Geometry check sheet. Reference: the model listing, model coordinates, mm. A direction names the side the tool comes from. Give positions to 0.01 mm unless a question says otherwise; leave off trailing zeros. Order: outer loops, then holes, each group sorted by start corner. A loop starts at its lowest first (then second) coordinate and runs counter-clockwise, first axis right, second up. Notation, with made-up numbers: M 73,5.5 L 93,5.5 A23 cw 93,43.5 Z; hole C 63.5,-26.5 d7. An arc over 180 degrees is marked long. Put each result on its own line as item: value. Start each with the question number.
Q1. Material ranges on L1, parallel to X at y = 17.75, z = 20; L2, parallel to Y at x = 45, z = 7; L3, parallel to Z at x = 37.5, y = 19, recorded low to high.
Q2. Section check A-A on y = 18. Record the cut outline in (x, z).
Q3. Section check C-C on z = -14.5. Record the cut outline in (x, y).
Q4. Mould release check, pull along Y, two halves, no side actions. Record for faces 4 (the cylindrical face through (8.628, 14.435, -21.014)), 5 (the flat face through (26, 24.7, -11)), 6 (the flat face through (24, 3, 32)): +Y half, -Y half, draft (parallel to the pull), parting line (faces both ways), or undercut.
Q5. Section check B-B on x = 22.5. Record the cut outline in (y, z).
Q6. Access from +Z, -Z, +X, -X, +Y, -Y to the whole of each face (thin tool, end or side, straight path). Record for faces 1 (the flat face through (3.4, 13, 17)), 2 (the flat face through (25, 1.4, 17)), 3 (the flat face through (49.4, 13, 17)).
Q7. Section check D-D on y = 12.7. Record the cut outline in (x, z), then the cut area to 3 significant figures.
Q8. Go/stop test with flat-tipped pins: pin 1 (24 mm diameter, centred on x = 19.5, z = 23, fed in from -Y); pin 2 (24 mm diameter, centred on x = 27.5, z = -9.5, fed in from +Y); pin 3 (7 mm diameter, centred on y = 15.5, z = 23.5, fed in from -X); pin 4 (10 mm diameter, centred on x = 26, z = -7, fed in from -Y). Record where each tip stops, or that it passes through.
Autodesk Inventor part; units mm, degrees
ref_plane "YZ Plane" through (0, 0, 0) normal (1, 0, 0) x (0, 1, 0)
ref_plane "XZ Plane" through (0, 0, 0) normal (0, 1, 0) x (-1, 0, 0)
ref_plane "XY Plane" through (0, 0, 0) normal (0, 0, 1) x (1, 0, 0)
sketch "Boceto1" plane through (0, 0, 0) normal (0, 0, 1) x (1, 0, 0)
  line L0 (0, 0) -> (50.8, 0)
  line L1 (50.8, 0) -> (50.8, 25.4)
  line L2 (50.8, 25.4) -> (0, 25.4)
  line L3 (0, 25.4) -> (0, 0)
  dimension "d0" = 50.8
  dimension "d1" = 25.4
extrude "Extrusión1" add sketch "Boceto1" along normal blind 2
sketch "Boceto2" plane through (0, 0, 2) normal (0, 0, 1) x (1, 0, 0)
  line L0 (1.4, 1.4) -> (49.4, 1.4)
  line L1 (49.4, 1.4) -> (49.4, 24)
  line L2 (49.4, 24) -> (1.4, 24)
  line L3 (1.4, 24) -> (1.4, 1.4)
  line L4 (0, 25.4) -> (0, 0)
  line L5 (0, 0) -> (50.8, 0)
  line L6 (50.8, 25.4) -> (0, 25.4)
  line L7 (50.8, 0) -> (50.8, 25.4)
  line L8 (3.4, 3.4) -> (47.4, 3.4)
  line L9 (47.4, 3.4) -> (47.4, 22)
  line L10 (47.4, 22) -> (3.4, 22)
  line L11 (3.4, 22) -> (3.4, 3.4)
  dimension "d4" = 1.4
  dimension "d5" = 1.4
  dimension "d6" = 1.4
  dimension "d7" = 1.4
  dimension "d8" = 2
  dimension "d9" = 2
  dimension "d10" = 2
  dimension "d11" = 2
extrude "Extrusión2" add sketch "Boceto2" along normal blind 30 contours L3 L2 L1 L0
sketch "Boceto3" plane through (50.8, 0, 0) normal (1, 0, 0) x (0, 0, -1)
  line L0 (0, 0) -> (0, 25.4)
  line L1 (0, 0.7) -> (22, 0.7)
  line L2 (22, 0.7) -> (22, 24.7)
  line L3 (22, 24.7) -> (0, 24.7)
  line L4 (0, 24.7) -> (0, 0.7)
  line L5 (0, 25.4) -> (-2, 25.4)
  line L6 (0, 0) -> (-2, 0)
  line L7 (0, 2.7) -> (20, 2.7)
  line L8 (20, 2.7) -> (20, 22.7)
  line L9 (20, 22.7) -> (0, 22.7)
  line L10 (0, 22.7) -> (0, 2.7)
  point P0 (-1, 25.4)
  point P1 (0, 24.7)
  point P2 (0, 22.7)
  point P3 (0, 2.7)
  point P4 (0, 0.7)
  dimension "d16" = 24
  dimension "d17" = 25.4
  dimension "d18" = 0.7
  dimension "d19" = 0.7
  dimension "d20" = 22
  dimension "d21" = 0
  dimension "d22" = 2
  dimension "d23" = 2
  dimension "d24" = 2
  dimension "d25" = 20
  dimension "d26" = 20
extrude "Extrusión3" add sketch "Boceto3" against normal up to surface (50.8 mm away) contours L0 L7 L8 L9 L3 L2 L1
sketch "Boceto4" plane through (50.8, 0.7, -22) normal (0, 0, -1) x (-1, 0, 0)
  circle A0 centre (8.4, 12) radius 1.75
  circle A1 centre (25.4, 12) radius 1.75
  circle A2 centre (42.4, 12) radius 1.75
  line L0 (50.8, 0) -> (50.8, 24)
  line L1 (0, 0) -> (0, 24)
  line L2 (0, 0) -> (50.8, 0)
  line L3 (0, 24) -> (50.8, 24)
  point P0 (50.8, -0.7)
  dimension "d29" = 3.5
  dimension "d30" = 3.5
  dimension "d31" = 3.5
  dimension "d32" = 17
  dimension "d33" = 17
  dimension "d34" = 50.8
  dimension "d39" = 24
  dimension "d40" = 12
  dimension "d41" = 12
  dimension "d42" = 12
  dimension "d43" = 12
  dimension "d44" = 12
  dimension "d45" = 25.4
  dimension "d46" = 8.4
extrude "Extrusión4" cut sketch "Boceto4" against normal up to surface (2 mm away) contours A0 | A1 | A2
properties part number "Tapa 51mm"
Results found:
1. L1: x = 1.4 to 3.4, 47.4 to 49.4
1. L2: y = 1.4 to 3.4, 22 to 24
1. L3: z = -22 to -20, 0 to 2
2. outline: M 0,-22 L 50.8,-22 L 50.8,-20 L 0,-20 Z; M 0,0 L 50.8,0 L 50.8,2 L 49.4,2 L 49.4,32 L 47.4,32 L 47.4,2 L 3.4,2 L 3.4,32 L 1.4,32 L 1.4,2 L 0,2 Z
3. outline: M 0,0.7 L 50.8,0.7 L 50.8,2.7 L 0,2.7 Z; M 0,22.7 L 50.8,22.7 L 50.8,24.7 L 0,24.7 Z
4. face 4: undercut
4. face 5: +Y half
4. face 6: draft
5. outline: M 0,0 L 0.7,0 L 0.7,-22 L 24.7,-22 L 24.7,0 L 25.4,0 L 25.4,2 L 24,2 L 24,32 L 22,32 L 22,2 L 3.4,2 L 3.4,32 L 1.4,32 L 1.4,2 L 0,2 Z; hole M 2.7,-20 L 22.7,-20 L 22.7,0 L 2.7,0 Z
6. face 1: +Z
6. face 2: +Z, +X, -X, -Y
6. face 3: +Z, +X, +Y, -Y
7. outline: M 0,-22 L 6.65,-22 L 6.65,-20 L 0,-20 Z; M 0,0 L 50.8,0 L 50.8,2 L 49.4,2 L 49.4,32 L 47.4,32 L 47.4,2 L 3.4,2 L 3.4,32 L 1.4,32 L 1.4,2 L 0,2 Z; M 10.15,-22 L 23.65,-22 L 23.65,-20 L 10.15,-20 Z; M 27.15,-22 L 40.65,-22 L 40.65,-20 L 27.15,-20 Z; M 44.15,-22 L 50.8,-22 L 50.8,-20 L 44.15,-20 Z
7. area: 302 mm^2
8. pin 1: stops at y = 1.4
8. pin 2: stops at y = 25.4
8. pin 3: stops at x = 1.4
8. pin 4: stops at y = 0.7
